Here's how the part is built. I have some questions about the finished solid (model axes, mm). A direction names the side the tool comes from. Round coordinates to 2 decimals unless told otherwise and drop trailing zeros. Loops run counter-clockwise (first coordinate to the right, second up) from the corner with the lowest first, then second, coordinate; pieces in that order, holes last. Notation, with made-up numbers: (-29, 88) -> (-14, 88) arc R8 cw to (-14, 92) -> close; hole circle Ø5 at (86.25, 23). An arc over 180 degrees is marked (long way). One line per item, written item: value. Start each with the question number.
```python
from build123d import *

# Parameters (mm, degrees)
ESQUISSE1_R             = 15.75
BOSS_EXTRU_1_DEPTH      = 5
ESQUISSE2_W             = 5.5
ESQUISSE2_H             = 2.985070052
BOSS_EXTRU_2_DEPTH      = 2.7
ESQUISSE3_R             = 1.75
ESQUISSE3_R_2           = 2.75
ESQUISSE3_R_3           = 3.1
ENL_V_MAT_EXTRU_1_DEPTH = 6
ESQUISSE4_W             = 7.942495838
ESQUISSE4_H             = 7.71802451
ENL_V_MAT_EXTRU_2_DEPTH = 6
ESQUISSE5_W             = 8
ESQUISSE5_H             = 5.5
ENL_V_MAT_EXTRU_3_DEPTH = 6


with BuildPart() as part:
    # Esquisse1 → Boss.-Extru.1 (new body)
    with BuildSketch(Plane.XY):
        Circle(ESQUISSE1_R)
    extrude(amount=BOSS_EXTRU_1_DEPTH)

    # Esquisse2 → Boss.-Extru.2 (add)
    with BuildSketch(Plane(origin=(0, 0, 0), x_dir=(-1, 0, 0), z_dir=(0, 0, -1))):
        with Locations((0, -15.007464974)):
            Rectangle(ESQUISSE2_W, ESQUISSE2_H)
    extrude(amount=-BOSS_EXTRU_2_DEPTH)

    # Esquisse3 → Enlèv. mat.-Extru.1 (cut, through all)
    with BuildSketch(Plane.XY.offset(5)):
        with Locations((0, 14.5)):
            Circle(ESQUISSE3_R)
        with Locations((9.5, 0)):
            Circle(ESQUISSE3_R_2)
        with Locations((-9.5, 0)):
            Circle(ESQUISSE3_R_2)
        with Locations((0, -9.5)):
            Circle(ESQUISSE3_R_3)
    extrude(amount=-ENL_V_MAT_EXTRU_1_DEPTH, mode=Mode.SUBTRACT)

    # Esquisse4 → Enlèv. mat.-Extru.2 (cut, through all)
    with BuildSketch(Plane.XY.offset(5)):
        with Locations((-10.275426072, -10.574276969)):
            Rectangle(ESQUISSE4_W, ESQUISSE4_H)
    enl_v_mat_extru_2 = extrude(amount=-ENL_V_MAT_EXTRU_2_DEPTH, mode=Mode.SUBTRACT)

    # Symétrie1: Enlèv. mat.-Extru.2 across plane
    add(enl_v_mat_extru_2.mirror(Plane(origin=(0, 0, 0), x_dir=(0, 0, 1), z_dir=(1, 0, 0))), mode=Mode.SUBTRACT)

    # Esquisse5 → Enlèv. mat.-Extru.3 (cut, through all)
    with BuildSketch(Plane.XY.offset(5)):
        with Locations((0, 5.75)):
            Rectangle(ESQUISSE5_W, ESQUISSE5_H)
    extrude(amount=-ENL_V_MAT_EXTRU_3_DEPTH, mode=Mode.SUBTRACT)


solid = part.part
```
Q1. I want a section at D-D on y = -9.5. Please give me the cut outline in (x, z).
Q2. Will these pins go through, and if not, where does the flat tip stop? P1, Ø3, axis at y = 9.5, z = 4, coming from the +X side; P2, Ø2.5, axis at x = 9.5, z = 2, coming from the -Y side; P3, Ø2, axis at x = 5.5, z = 3.5, coming from the -Y side.
Q3. If I drill on line 1 along Y through (x, z) = (0, 3.5); line 2 along X through (y, z) = (1, 4.1); line 3 along X through (y, z) = (-1.5, 4.5), over which ranges is the centre line in solid material (lowest first)?
Q4. Which directions (+Z, -Z, +X, -X, +Y, -Y) give clear straight access to the entire face, cutting with the end or side of a thin tool? Please do faces 1 (the flat face through (0, -16.5, 1)), 2 (the flat face through (10, -6.715, 3)), 3 (the flat face through (0, 8.5, 3)), 4 (the flat face through (0, 0, 5)), 5 (the flat face through (-2.75, -16, 1)).
Q5. I want a section at C-C on x = 0. Please give me the cut outline in (y, z).
Q6. If we mould it in two halves opening along X, with no side actions, what happens to faces 6 (the flat face through (0, 0, 0)), 7 (the cylindrical face through (-0.09, -15.75, 3.02)), 8 (the flat face through (4, 6, 3))? For each: released by +X, released by -X, zero draft, split by the parting line, or undercut.
Q7. I want a section at B-B on z = 4.2. Please give me the cut outline in (x, y), plus the area to 3 significant figures.
Q8. I want a section at A-A on y = 0. Please give me the cut outline in (x, z).
Answers below:
1. outline: (-6.3, 0) -> (-3.1, 0) -> (-3.1, 5) -> (-6.3, 5) -> close; (3.1, 0) -> (6.3, 0) -> (6.3, 5) -> (3.1, 5) -> close
2. P1: stops at x = 13.57
2. P2: stops at y = -6.72
2. P3: stops at y = -15.09
3. line 1: y = -15.75 to -12.6, -6.4 to 3, 8.5 to 12.75
3. line 2: x = -15.72 to -12.06, -6.94 to 6.94, 12.06 to 15.72
3. line 3: x = -15.68 to -11.8, -7.2 to 7.2, 11.8 to 15.68
4. face 1: +Z, -Z, +X, -X, -Y
4. face 2: +Z, -Z, +X, -Y
4. face 3: +Z, -Z
4. face 4: +Z, +X, -X, +Y, -Y
4. face 5: +Z, -Z, -X, -Y
5. outline: (-16.5, 0) -> (-12.6, 0) -> (-12.6, 5) -> (-15.75, 5) -> (-15.75, 2.7) -> (-16.5, 2.7) -> close; (-6.4, 0) -> (3, 0) -> (3, 5) -> (-6.4, 5) -> close; (8.5, 0) -> (12.75, 0) -> (12.75, 5) -> (8.5, 5) -> close
6. face 6: zero draft
6. face 7: split by the parting line
6. face 8: undercut
7. outline: (-14.25, -6.72) -> (-6.3, -6.72) -> (-6.3, -14.43) arc R15.75 ccw to (6.3, -14.43) -> (6.3, -6.72) -> (14.25, -6.72) arc R15.75 ccw to (1.28, 15.7) arc R1.75 cw (long way) to (-1.28, 15.7) arc R15.75 ccw to start; hole circle Ø5.5 at (-9.5, 0); hole (-4, 3) -> (4, 3) -> (4, 8.5) -> (-4, 8.5) -> close; hole circle Ø6.2 at (0, -9.5); hole circle Ø5.5 at (9.5, 0)
7. area: 573 mm^2
8. outline: (-15.75, 0) -> (-12.25, 0) -> (-12.25, 5) -> (-15.75, 5) -> close; (-6.75, 0) -> (6.75, 0) -> (6.75, 5) -> (-6.75, 5) -> close; (12.25, 0) -> (15.75, 0) -> (15.75, 5) -> (12.25, 5) -> close
